The model under review builds one solid part; all positions refer to its coordinate system, in mm. Give positions to 0.01 mm unless a question says otherwise; leave off trailing zeros. Write each loop counter-clockwise with the first axis right and the second up, starting at its lowest first coordinate (ties: lowest second). Pieces come first, ordered by that corner, then holes. Notation, with made-up numbers: (-25.75, -20.75) - (-11.75, -20.75) arc R10 cw to (-11.75, -11.75) - close; hole circle Ø5 at (3, 68.5). An arc over 180 degrees is marked (long way). Write item = value, one per line.
```python
from build123d import *

# Parameters (mm, degrees)
F0_W     = 52
F0_H     = 158.4
F0_W_2   = 5.9
F0_H_2   = 42
F0_W_3   = 21
F0_H_3   = 5.9
F0_W_4   = 8.76
F0_H_4   = 12
F1_DEPTH = 5.9


with BuildPart() as f1:
    # F0 (on Right) → F1 (new body)
    with BuildSketch(Plane.YZ):
        Rectangle(F0_W, F0_H)
        with Locations((-17, -40.2)):
            Rectangle(F0_W_2, F0_H_2, mode=Mode.SUBTRACT)
        with Locations((-9.45, -70.15)):
            Rectangle(F0_W_3, F0_H_3, mode=Mode.SUBTRACT)
        with Locations((15.33, -61.2)):
            Rectangle(F0_W_4, F0_H_4, mode=Mode.SUBTRACT)
        with Locations((-17, 40.2)):
            Rectangle(F0_W_2, F0_H_2, mode=Mode.SUBTRACT)
        with Locations((-9.45, 70.15)):
            Rectangle(F0_W_3, F0_H_3, mode=Mode.SUBTRACT)
        with Locations((15.33, 61.2)):
            Rectangle(F0_W_4, F0_H_4, mode=Mode.SUBTRACT)
    extrude(amount=F1_DEPTH)


solid = f1.part
```
1. Take a section at B-B on z = 45.5. Give the boundary of the cut face in (x, y), and give its area (3 significant figures).
Findings below:
outline = (0, -26) - (5.9, -26) - (5.9, -19.95) - (0, -19.95) - close; (0, -14.05) - (5.9, -14.05) - (5.9, 26) - (0, 26) - close
area = 272 mm²
2. Draft analysis for pull direction Y (two halves, no side actions). For faces 1 (the flat face through (3, 15, -67.2)), 2 (the flat face through (3, 26, -1)), 3 (the flat face through (0, 0, 1)), state which applies: +Y half, -Y half, draft (parallel to the pull), parting line (faces both ways), or undercut.
Findings below:
face_1 = undercut
face_2 = +Y half
face_3 = draft
3. Take a section at A-A on y = -9.5. Give the boundary of the cut face in (x, z).
Findings below:
outline = (0, -79.2) - (5.9, -79.2) - (5.9, -73.1) - (0, -73.1) - close; (0, -67.2) - (5.9, -67.2) - (5.9, 67.2) - (0, 67.2) - close; (0, 73.1) - (5.9, 73.1) - (5.9, 79.2) - (0, 79.2) - close
4. For line 1 (Z direction, x = 2.35, y = 11); line 2 (Z direction, x = 2.85, y = -2.5); line 3 (Z direction, x = 1.4, y = -19), list the stretches that pass through material, from the lowest coordinate up. Write a range as from..to.
Findings below:
line_1 = -79.2..-67.2, -55.2..55.2, 67.2..79.2
line_2 = -79.2..-73.1, -67.2..67.2, 73.1..79.2
line_3 = -79.2..-73.1, -67.2..-61.2, -19.2..19.2, 61.2..67.2, 73.1..79.2
5. Take a section at C-C on x = 1.3. Give the boundary of the cut face in (y, z).
Findings below:
outline = (-26, -79.2) - (26, -79.2) - (26, 79.2) - (-26, 79.2) - close; hole (-19.95, -73.1) - (1.05, -73.1) - (1.05, -67.2) - (-19.95, -67.2) - close; hole (-19.95, -61.2) - (-14.05, -61.2) - (-14.05, -19.2) - (-19.95, -19.2) - close; hole (-19.95, 19.2) - (-14.05, 19.2) - (-14.05, 61.2) - (-19.95, 61.2) - close; hole (-19.95, 67.2) - (1.05, 67.2) - (1.05, 73.1) - (-19.95, 73.1) - close; hole (10.95, -67.2) - (19.71, -67.2) - (19.71, -55.2) - (10.95, -55.2) - close; hole (10.95, 55.2) - (19.71, 55.2) - (19.71, 67.2) - (10.95, 67.2) - close
6. Insertion check: P1, Ø6, axis at y = 5, z = -33.5, coming from the -X side. The pin has a flat end and moves straight along its axis. Give the tip position at first contact, or say it passes through.
Findings below:
P1 = 0
7. Take a section at D-D on z = 69. Give the boundary of the cut face in (x, y), and give its area (3 significant figures).
Findings below:
outline = (0, -26) - (5.9, -26) - (5.9, -19.95) - (0, -19.95) - close; (0, 1.05) - (5.9, 1.05) - (5.9, 26) - (0, 26) - close
area = 183 mm²
